from build123d import *

# Parameters (mm, degrees)
BOSS_EXTRUDE1_DEPTH = 3.5


with BuildPart() as part:
    # Sketch1 → Boss-Extrude1 (new, symmetric)
    with BuildSketch(Plane(origin=(0, 0, 0), x_dir=(0, 0, -1), z_dir=(1, 0, 0))):
        with BuildLine():
            Line((0, 15), (0, -15))
            ThreePointArc((0, -15), (16.267428438, -28.732571562), (30, -45))
            ThreePointArc((30, -45), (43.342526908, -57.873390661), (60.45856181, -65))
            ThreePointArc((60.45856181, -65), (67.649976256, -62.944872105), (70, -55.84435235))
            ThreePointArc((70, -55.84435235), (61.345746077, -30.825000689), (45, -10))
            ThreePointArc((45, -10), (40.583973737, 0), (45, 10))
            ThreePointArc((45, 10), (61.345746077, 30.825000689), (70, 55.84435235))
            ThreePointArc((70, 55.84435235), (67.649976256, 62.944872105), (60.45856181, 65))
            ThreePointArc((60.45856181, 65), (43.342526908, 57.873390661), (30, 45))
            ThreePointArc((30, 45), (16.267428438, 28.732571562), (0, 15))
        make_face()
    extrude(amount=BOSS_EXTRUDE1_DEPTH, both=True)


solid = part.part
The listing builds one solid part. Answer for the finished solid, in the listing's coordinates (mm). A direction names the side the tool comes from. Coordinates: 2 decimals unless noted, no trailing zeros. Loops run counter-clockwise (first coordinate to the right, second up) from the corner with the lowest first, then second, coordinate; pieces in that order, holes last.
1) Find section B-B on x = -0.75. Write down the section's boundary in (y, z).
2) A tool of negligible diameter and unlimited length cuts with its end or side. For faces 4 (the face through (0.049, -57.73, -43.125)), 5 (the face through (0.049, 30.499, -61.167)), from which of +Z, -Z, +X, -X, +Y, -Y can it reach the whole face along a straight path? Write none if from no direction.
3) Determine the mould class of faces 1 (the face through (0.05, -31.15, -61.52)), 2 (the face through (3.5, 1, -35)), 3 (the face through (0.049, 58.016, -43.561)) for opening direction Y: pulls with the +Y half, pulls with the -Y half, needs draft (parallel to the pull), parting line crosses it, or undercut.
4) Find the intervals of material crossed by L1, parallel to Y at x = 2.75, z = -53.5 (3 decimals); L2, parallel to Y at x = -3, z = -44; L3, parallel to Y at x = -2.25, z = -12.5, in increasing order.
5) Find section A-A on z = -64. Write down the section's boundary in (x, y).
6) Find section C-C on z = -47. Write down the section's boundary in (x, y), then the cut area to 3 significant figures.
7) Flat-ended cylindrical pins translate along their axes: pin 1 Ø1.5 at (x, z) = (-1, -53.5) entering from -Y; pin 2 Ø1 at (x, z) = (-0.5, -15.5) entering from -Y. Find the tip coordinate at first contact, or state that the pin passes through.
8) Find section D-D on y = -27.5. Write down the section's boundary in (x, z), then the cut area to 3 significant figures.
Values:
1. outline: (-65, -60.46) arc R8 ccw to (-55.84, -70) arc R80 ccw to (-10, -45) arc R13.53 cw to (10, -45) arc R80 ccw to (55.84, -70) arc R8 ccw to (65, -60.46) arc R50 ccw to (45, -30) arc R126.43 cw to (15, 0) - (-15, 0) arc R126.43 cw to (-45, -30) arc R50 ccw to start
2. face 4: +Z, +X, -X, -Y
2. face 5: -Z, +X, -X
3. face 1: undercut
3. face 2: needs draft
3. face 3: pulls with the +Y half
4. L1: y = -62.995 to -19.051, 19.051 to 62.995
4. L2: y = -58.3 to -8.99, 8.99 to 58.3
4. L3: y = -25.12 to 25.12
5. outline: (-3.5, -64.95) - (3.5, -64.95) - (3.5, -36.16) - (-3.5, -36.16) - close; (-3.5, 36.16) - (3.5, 36.16) - (3.5, 64.95) - (-3.5, 64.95) - close
6. outline: (-3.5, -60.06) - (3.5, -60.06) - (3.5, -11.89) - (-3.5, -11.89) - close; (-3.5, 11.89) - (3.5, 11.89) - (3.5, 60.06) - (-3.5, 60.06) - close
6. area: 674 mm2
7. pin 1: stops at y = -63.26
7. pin 2: stops at y = -28.47
8. outline: (-3.5, -59.43) - (3.5, -59.43) - (3.5, -15.02) - (-3.5, -15.02) - close
8. area: 311 mm2
